from build123d import *

# Parameters (mm, degrees)
SKETCH1_R           = 23
SKETCH1_R_2         = 21
BOSS_EXTRUDE1_DEPTH = 25
SKETCH2_R           = 32.5
SKETCH2_R_2         = 23
BOSS_EXTRUDE2_DEPTH = 2
FILLET1_R           = 10
FILLET2_R           = 3


with BuildPart() as part:
    # Sketch1 → Boss-Extrude1 (new body)
    with BuildSketch(Plane(origin=(0, 0, 0), x_dir=(1, 0, 0), z_dir=(0, 1, 0))):
        with Locations(Location((0, 0, 0), (0, 0, 270))):
            Circle(SKETCH1_R)
        with Locations(Location((0, 0, 0), (0, 0, 270))):
            Circle(SKETCH1_R_2, mode=Mode.SUBTRACT)
    extrude(amount=BOSS_EXTRUDE1_DEPTH)

    # Sketch2 → Boss-Extrude2 (add)
    with BuildSketch(Plane(origin=(0, 0, 0), x_dir=(1, 0, 0), z_dir=(0, 1, 0))):
        with Locations(Location((0, 0, 0), (0, 0, 270))):
            Circle(SKETCH2_R)
        with Locations(Location((0, 0, 0), (0, 0, 270))):
            Circle(SKETCH2_R_2, mode=Mode.SUBTRACT)
    extrude(amount=BOSS_EXTRUDE2_DEPTH)

    # Fillet1
    # the kernel refuses this fillet: 10 mm, written as the material it adds along each edge
    with BuildSketch(Plane(origin=(0, 2, 0), x_dir=(-1.8e-16, 0, 1), z_dir=(-1, 0, -1.8e-16))) as fillet1_piece_1:
        with BuildLine():
            CenterArc((33, 9.98749217771909), FILLET1_R, 180, 87.13401601740111)
            Line((32.5, 1.78e-15), (32.49, -0.19974984355438008))
            ThreePointArc((32.49, -0.19974984355438008), (27.75, -0.19999999999999996), (23, -0.19999999999999996))
            Line((23, -0.19999999999999996), (22.8, 0))
            Line((22.8, 0), (22.8, 9.98749217771909))
            Line((22.8, 9.98749217771909), (23, 9.98749217771909))
        make_face()
    revolve(axis=Axis((0, 2, 0), (0, 1, 0)))

    # Fillet2
    fillet2_edges = [part.edges().sort_by_distance(p)[0] for p in [
        (6.43e-15, 0, -21),
    ]]
    fillet(fillet2_edges, radius=FILLET2_R)


solid = part.part
Check sheet for the modelled part. Datum: model origin and axes. Units: mm. Round coordinates to 2 decimals unless told otherwise and drop trailing zeros. Write each loop counter-clockwise with the first axis right and the second up, starting at its lowest first coordinate (ties: lowest second). Pieces come first, ordered by that corner, then holes. Notation, with made-up numbers: (22, 70.5) -> (27, 70.5) arc R23 cw to (27, 106.5) -> close; hole circle Ø8 at (24.25, 28.25). An arc over 180 degrees is marked (long way). Answer as CSV lines item,"result". Start each with the question number.
1) Section check C-C on y = 18.75. Enter the section's corners in (x, z).
2) Section check A-A on x = 0. Enter the section's corners in (y, z).
3) Release check for a two-part mould opening along Z. For faces 1 (the cylindrical face through (6.31, 13.85, 20.03)), 2 (the cylindrical face through (19.394, 18.403, 12.365)), 3 (the flat face through (-24, 0, -3)) record: pulls with the +Z half, pulls with the -Z half, needs draft (parallel to the pull), parting line crosses it, or undercut.
4) Section check B-B on z = 0. Enter the section's corners in (x, y).
5) Material ranges on line 1 (X direction, y = 16, z = 0); line 2 (X direction, y = 9.5, z = 0); line 3 (Y direction, x = 19, z = 26), recorded low to high. Write a range as from..to.
6) Go/stop test with flat-tipped pins: P1, Ø2, axis at y = 5, z = 15.5, coming from the -X side; P2, Ø1, axis at x = -19.5, y = 12, coming from the -Z side; P3, Ø1.5, axis at y = 20.5, z = 20.5, coming from the +X side; P4, Ø5, axis at x = -12.5, z = -11.5, coming from the -Y side. Record where each tip stops, or that it passes through.
Found:
1,outline,"circle Ø46 at (0, 0); hole circle Ø42 at (0, 0)"
2,outline,"(0, -32.5) -> (2, -32.5) arc R10 cw to (11.99, -23) -> (25, -23) -> (25, -21) -> (3, -21) arc R3 ccw to (0, -24) -> close; (0, 24) arc R3 ccw to (3, 21) -> (25, 21) -> (25, 23) -> (11.99, 23) arc R10 cw to (2, 32.5) -> (0, 32.5) -> close"
3,face 1,"undercut"
3,face 2,"parting line crosses it"
3,face 3,"needs draft"
4,outline,"(-32.5, 0) -> (-24, 0) arc R3 ccw to (-21, 3) -> (-21, 25) -> (-23, 25) -> (-23, 11.99) arc R10 cw to (-32.5, 2) -> close; (21, 3) arc R3 ccw to (24, 0) -> (32.5, 0) -> (32.5, 2) arc R10 cw to (23, 11.99) -> (23, 25) -> (21, 25) -> close"
5,line 1,"x = -23..-21, 21..23"
5,line 2,"x = -23.31..-21, 21..23.31"
5,line 3,"y = 0..2.02"
6,P1,"stops at x = -22.23"
6,P2,"stops at z = -12.96"
6,P3,"stops at x = 11.79"
6,P4,"passes through"
